For this review, take the finished solid that the model builds, in its own axes (mm). A direction names the side the tool comes from. Coordinates: 2 decimals unless noted, no trailing zeros. Loops run counter-clockwise (first coordinate to the right, second up) from the corner with the lowest first, then second, coordinate; pieces in that order, holes last. Notation, with made-up numbers: (-8.5, 1.25) - (21.5, 1.25) arc R14 cw to (21.5, 24.25) - close; hole circle Ø9 at (62.5, -38.75). An arc over 180 degrees is marked (long way). Use one line per item in the form item = value. Start each with the question number.
1. Add section B-B on y = 56. Give the boundary of the cut face in (x, z).
2. To check wall thickness, follow probe 1 along Z at (x, y) = (-44, 56.05). State the ranges of the line that lie inside material, in increasing order.
3. Add section C-C on x = -80.5. Give the boundary of the cut face in (y, z), and give its area (3 significant figures).
4. For pin 1 Ø1 at (y, z) = (57, 10) entering from -X; pin 2 Ø0.5 at (x, z) = (-79, 11) entering from -Y; pin 3 Ø0.5 at (y, z) = (54.5, 13) entering from +X, all flat-tipped, find the tip position at first contact; note any pin that passes through.
5. Add section A-A on z = 12.5. Count the separate pieces of the cut face and the enclosed holes in it, and give its area (3 significant figures).
6. Machinability: for faces 4 (the face through (-55.684, 57, 11)), 5 (the face through (-48.5, 54.055, 11.5)), 6 (the face through (-46, 57.495, 11)), which of the approach directions +Z, -Z, +X, -X, +Y, -Y give a long, thin tool a straight path to every point of the face, cutting with its end or side? Answer none if there is none.
7. Draft analysis for pull direction Y (two halves, no side actions). For faces 1 (the face through (-81.5, 54.955, 11.5)), 2 (the face through (-66, 54.055, 11)), 3 (the face through (-73.464, 57, 11)), state which applies: +Y half, -Y half, draft (parallel to the pull), parting line (faces both ways), or undercut.
```python
from build123d import *

# Parameters (mm, degrees)
SKETCH_1_W      = 51
SKETCH_1_H      = 5
EXTRUDE_1_DEPTH = 8.5
SKETCH_3_W      = 0.9
SKETCH_3_H      = 0.9
EXTRUDE_2_DEPTH = 6


with BuildPart() as part:
    # 草图1 → 凸台-拉伸1 (new body)
    with BuildSketch(Plane.XY):
        with Locations((-62.234353046, 55.774690545)):
            Rectangle(SKETCH_1_W, SKETCH_1_H)
    extrude(amount=EXTRUDE_1_DEPTH)

    # 草图3 → 凸台-拉伸2 (add)
    with BuildSketch(Plane.XY.offset(8.5)):
        with Locations((-84.074353046, 57.044690545)):
            Rectangle(SKETCH_3_W, SKETCH_3_H)
        with Locations((-86.614353046, 57.044690545)):
            Rectangle(SKETCH_3_W, SKETCH_3_H)
        with Locations((-81.534353046, 57.044690545)):
            Rectangle(SKETCH_3_W, SKETCH_3_H)
        with Locations((-78.994353046, 57.044690545)):
            Rectangle(SKETCH_3_W, SKETCH_3_H)
        with Locations((-76.454353046, 57.044690545)):
            Rectangle(SKETCH_3_W, SKETCH_3_H)
        with Locations((-73.914353046, 57.044690545)):
            Rectangle(SKETCH_3_W, SKETCH_3_H)
        with Locations((-71.374353046, 57.044690545)):
            Rectangle(SKETCH_3_W, SKETCH_3_H)
        with Locations((-68.834353046, 57.044690545)):
            Rectangle(SKETCH_3_W, SKETCH_3_H)
        with Locations((-66.294353046, 57.044690545)):
            Rectangle(SKETCH_3_W, SKETCH_3_H)
        with Locations((-63.754353046, 57.044690545)):
            Rectangle(SKETCH_3_W, SKETCH_3_H)
        with Locations((-61.214353046, 57.044690545)):
            Rectangle(SKETCH_3_W, SKETCH_3_H)
        with Locations((-58.674353046, 57.044690545)):
            Rectangle(SKETCH_3_W, SKETCH_3_H)
        with Locations((-56.134353046, 57.044690545)):
            Rectangle(SKETCH_3_W, SKETCH_3_H)
        with Locations((-53.594353046, 57.044690545)):
            Rectangle(SKETCH_3_W, SKETCH_3_H)
        with Locations((-51.054353046, 57.044690545)):
            Rectangle(SKETCH_3_W, SKETCH_3_H)
        with Locations((-48.514353046, 57.044690545)):
            Rectangle(SKETCH_3_W, SKETCH_3_H)
        with Locations((-45.974353046, 57.044690545)):
            Rectangle(SKETCH_3_W, SKETCH_3_H)
        with Locations((-43.434353046, 57.044690545)):
            Rectangle(SKETCH_3_W, SKETCH_3_H)
        with Locations((-40.894353046, 57.044690545)):
            Rectangle(SKETCH_3_W, SKETCH_3_H)
        with Locations((-38.354353046, 57.044690545)):
            Rectangle(SKETCH_3_W, SKETCH_3_H)
        with Locations((-84.074353046, 54.504690545)):
            Rectangle(SKETCH_3_W, SKETCH_3_H)
        with Locations((-81.534353046, 54.504690545)):
            Rectangle(SKETCH_3_W, SKETCH_3_H)
        with Locations((-78.994353046, 54.504690545)):
            Rectangle(SKETCH_3_W, SKETCH_3_H)
        with Locations((-76.454353046, 54.504690545)):
            Rectangle(SKETCH_3_W, SKETCH_3_H)
        with Locations((-73.914353046, 54.504690545)):
            Rectangle(SKETCH_3_W, SKETCH_3_H)
        with Locations((-71.374353046, 54.504690545)):
            Rectangle(SKETCH_3_W, SKETCH_3_H)
        with Locations((-68.834353046, 54.504690545)):
            Rectangle(SKETCH_3_W, SKETCH_3_H)
        with Locations((-66.294353046, 54.504690545)):
            Rectangle(SKETCH_3_W, SKETCH_3_H)
        with Locations((-63.754353046, 54.504690545)):
            Rectangle(SKETCH_3_W, SKETCH_3_H)
        with Locations((-61.214353046, 54.504690545)):
            Rectangle(SKETCH_3_W, SKETCH_3_H)
        with Locations((-58.674353046, 54.504690545)):
            Rectangle(SKETCH_3_W, SKETCH_3_H)
        with Locations((-56.134353046, 54.504690545)):
            Rectangle(SKETCH_3_W, SKETCH_3_H)
        with Locations((-53.594353046, 54.504690545)):
            Rectangle(SKETCH_3_W, SKETCH_3_H)
        with Locations((-51.054353046, 54.504690545)):
            Rectangle(SKETCH_3_W, SKETCH_3_H)
        with Locations((-48.514353046, 54.504690545)):
            Rectangle(SKETCH_3_W, SKETCH_3_H)
        with Locations((-45.974353046, 54.504690545)):
            Rectangle(SKETCH_3_W, SKETCH_3_H)
        with Locations((-43.434353046, 54.504690545)):
            Rectangle(SKETCH_3_W, SKETCH_3_H)
        with Locations((-40.894353046, 54.504690545)):
            Rectangle(SKETCH_3_W, SKETCH_3_H)
        with Locations((-38.354353046, 54.504690545)):
            Rectangle(SKETCH_3_W, SKETCH_3_H)
        with Locations((-86.614353046, 54.504690545)):
            Rectangle(SKETCH_3_W, SKETCH_3_H)
    extrude(amount=EXTRUDE_2_DEPTH)


solid = part.part
```
Conclusion:
q1.outline = (-87.73, 0) - (-36.73, 0) - (-36.73, 8.5) - (-87.73, 8.5) - close
q2.probe_1 = 0 to 8.5
q3.outline = (53.27, 0) - (58.27, 0) - (58.27, 8.5) - (53.27, 8.5) - close
q3.area = 42.5 mm^2
q4.pin_1 = -87.06
q4.pin_2 = 54.05
q4.pin_3 = -37.9
q5.separate_pieces = 40
q5.enclosed_holes = 0
q5.area = 32.4 mm^2
q6.face_4 = +Z, +Y, -Y
q6.face_5 = +Z, +X, -X, -Y
q6.face_6 = +Z, +X, -X, +Y
q7.face_1 = undercut
q7.face_2 = -Y half
q7.face_3 = draft
